from build123d import *

# Parameters (mm, degrees)
F1_DEPTH = 4
F2_R     = 1.775795
F3_DEPTH = 6.966509
F4_R     = 0.5


with BuildPart() as f1:
    # F0 (on Top) → F1 (new body, symmetric)
    with BuildSketch(Plane.XY):
        with BuildLine():
            Line((-33.881166, 2), (-33.881166, 0))
            Line((-33.881166, 0), (-14.881166, 0))
            Line((-14.881166, 0), (-14.881166, 14.3338))
            Line((-14.881166, 14.3338), (14.881166, 14.3338))
            Line((14.881166, 14.3338), (14.881166, -1.965509))
            Line((14.881166, -1.965509), (16.881166, -1.965509))
            ThreePointArc((16.881166, -1.965509), (19.002486, -1.08683), (19.881166, 1.034491))
            Line((19.881166, 1.034491), (19.881166, 16.3338))
            ThreePointArc((19.881166, 16.3338), (19.002486, 18.45512), (16.881166, 19.3338))
            Line((16.881166, 19.3338), (-16.881166, 19.3338))
            ThreePointArc((-16.881166, 19.3338), (-19.002486, 18.45512), (-19.881166, 16.3338))
            Line((-19.881166, 16.3338), (-19.881166, 8))
            ThreePointArc((-19.881166, 8), (-20.759845, 5.87868), (-22.881166, 5))
            Line((-22.881166, 5), (-30.881166, 5))
            ThreePointArc((-30.881166, 5), (-33.002486, 4.12132), (-33.881166, 2))
        make_face()
    extrude(amount=F1_DEPTH, both=True)

    # F2 (on face) → F3 (cut, through all)
    with BuildSketch(Plane(origin=(0, 5, 0), x_dir=(-1, 0, 0), z_dir=(0, 1, 0))):
        with Locations((26.881166, 0)):
            Circle(F2_R)
    extrude(amount=-F3_DEPTH, mode=Mode.SUBTRACT)

    # F4
    f4_edges = [f1.edges().sort_by_distance(p)[0] for p in [
        (-33.881166, 1, 4),
        (-24.381166, 0, 4),
        (-14.881166, 7.1669, 4),
        (0, 14.3338, 4),
        (14.881166, 6.184145, 4),
        (15.881166, -1.965509, 4),
        (19.002486, -1.08683, 4),
        (19.881166, 8.684145, 4),
        (19.002486, 18.45512, 4),
        (0, 19.3338, 4),
        (-19.002486, 18.45512, 4),
        (-19.881166, 12.1669, 4),
        (-20.759845, 5.87868, 4),
        (-26.881166, 5, 4),
        (-33.002486, 4.12132, 4),
        (-33.881166, 1, -4),
        (-24.381166, 0, -4),
        (-14.881166, 7.1669, -4),
        (0, 14.3338, -4),
        (14.881166, 6.184145, -4),
        (15.881166, -1.965509, -4),
        (19.002486, -1.08683, -4),
        (19.881166, 8.684145, -4),
        (19.002486, 18.45512, -4),
        (0, 19.3338, -4),
        (-19.002486, 18.45512, -4),
        (-19.881166, 12.1669, -4),
        (-20.759845, 5.87868, -4),
        (-26.881166, 5, -4),
        (-33.002486, 4.12132, -4),
    ]]
    fillet(f4_edges, radius=F4_R)


solid = f1.part
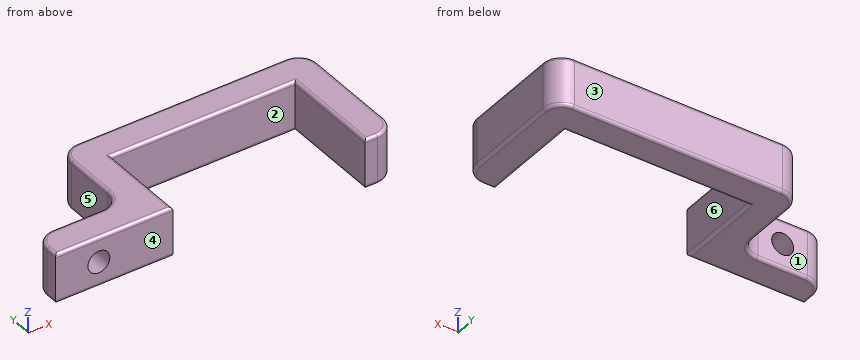
Part model, mm, in its own coordinate system. Face numbers are marked on the shaded views. A direction names the side the tool comes from. Give positions to 0.01 mm unless a question says otherwise; leave off trailing zeros. Order: outer loops, then holes, each group sorted by start corner. A loop starts at its lowest first (then second) coordinate and runs counter-clockwise, first axis right, second up. Notation, with made-up numbers: (82, 52.25) - (109, 52.25) arc R29 ccw to (109, 90.25) - close; hole circle Ø1 at (11, 35.25). An arc over 180 degrees is marked (long way). Use a Markdown table: item, result.
1) 3-axis set-ups, long thin cutter, end or side, ignore diameter. For the marked faces 1, 2 and 3: which of +Z, -Z, +X, -X, +Y, -Y reach the whole face in a straight line?
Checked values:
| item | result |
|---|---|
| face 1 | +Z, -Z, -X, +Y |
| face 2 | +Z, -Z, -Y |
| face 3 | +Z, -Z, +X, -X, +Y |
2) Two-plate mould, pull along X, no slides. Class the marked faces 4, 5 and 6: +X half, -X half, draft (parallel to the pull), parting line (faces both ways), or undercut.
Checked values:
| item | result |
|---|---|
| face 4 | draft |
| face 5 | -X half |
| face 6 | undercut |
3) Probe L1, parallel to X at y = 12.75, z = -3.5; L2, parallel to Y at x = -4, z = -0.25; L3, parallel to Y at x = -15, z = 2.5. List the from-to ranges inside material, lowest first. Write a range as from..to.
Checked values:
| item | result |
|---|---|
| L1 | -19.88..-14.88, 14.88..19.88 |
| L2 | 14.33..19.33 |
| L3 | 0..19.33 |
4) Saw through at B-B on x = 0. List the corners of the cut face in (y, z), plus the area to 3 significant figures.
Checked values:
| item | result |
|---|---|
| outline | (14.33, -3.5) arc R0.5 ccw to (14.83, -4) - (18.83, -4) arc R0.5 ccw to (19.33, -3.5) - (19.33, 3.5) arc R0.5 ccw to (18.83, 4) - (14.83, 4) arc R0.5 ccw to (14.33, 3.5) - close |
| area | 39.8 mm² |
5) Flat gauge pins, fed straight in: P1, Ø3.5, axis at x = -27.5, z = 1.5, coming from the +Y side; P2, Ø2, axis at y = 11.5, z = 3, coming from the -X side; P3, Ø1.5, axis at x = -2, z = -2.5, coming from the -Y side. Where does each tip first touch, or does it go through?
Checked values:
| item | result |
|---|---|
| P1 | y = 5 |
| P2 | x = -19.88 |
| P3 | y = 14.33 |
6) Saw through at A-A on z = 0. List the corners of the cut face in (x, y), plus the area to 3 significant figures.
Checked values:
| item | result |
|---|---|
| outline | (-33.88, 0) - (-28.66, 0) - (-28.66, 5) - (-30.88, 5) arc R3 ccw to (-33.88, 2) - close; (-25.11, 0) - (-14.88, 0) - (-14.88, 14.33) - (14.88, 14.33) - (14.88, -1.97) - (16.88, -1.97) arc R3 ccw to (19.88, 1.03) - (19.88, 16.33) arc R3 ccw to (16.88, 19.33) - (-16.88, 19.33) arc R3 ccw to (-19.88, 16.33) - (-19.88, 8) arc R3 cw to (-22.88, 5) - (-25.11, 5) - close |
| area | 398 mm² |
